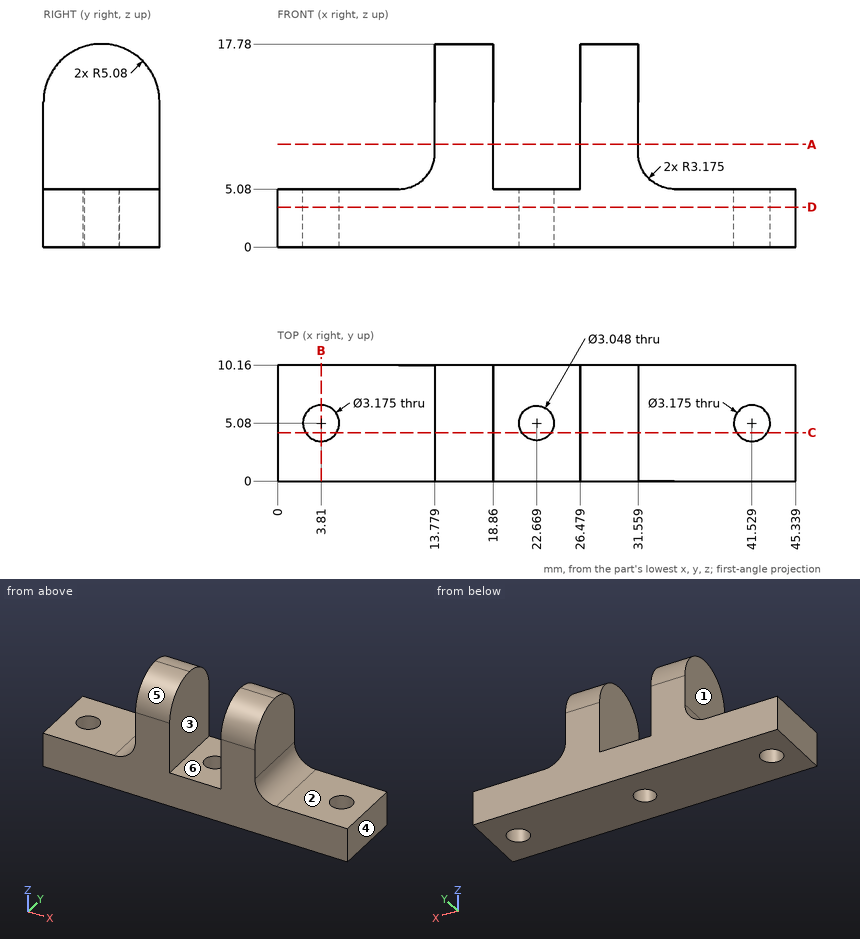
Here's the drawing with two shaded views (mm, measured from the low corner). I have some questions. A direction names the side the tool comes from. Give positions to 0.01 mm unless a question says otherwise; leave off trailing zeros. Loops run counter-clockwise (first coordinate to the right, second up) from the corner with the lowest first, then second, coordinate; pieces in that order, holes last. Notation, with made-up numbers: (2, -36.75) -> (48, -36.75) arc R11 cw to (48, -20.75) -> close; hole circle Ø1 at (-29, 67.25). An arc over 180 degrees is marked (long way). Answer as a JSON object with one key per item and string values. Group by question number.
Item 1: Imagine slicing it at C-C on y = 4.25. Give the number of separate pieces and of enclosed holes in the cut face.
Item 2: Thinking about a two-plate mould opening in X: for the marked faces 4, 5 and 6, which applies, pulls with the +X half, pulls with the -X half, needs draft (parallel to the pull), parting line crosses it, or undercut?
Item 3: I need wall thicknesses on L1, parallel to Y at x = 3.81, z = 3; L2, parallel to X at y = 6, z = 8; L3, parallel to X at y = 5.5, z = 3 (1 decimal). Which ranges of each line are inside material? Lowest first, please.
Item 4: Imagine slicing it at A-A on z = 9. Write out the boundary of the cut face in (x, y).
Item 5: Imagine slicing it at D-D on z = 3.5. Write out the boundary of the cut face in (x, y) (1 decimal).
Item 6: Will these pins go through, and if not, where does the flat tip stop? pin 1 (3.5 mm diameter, centred on x = 22.67, y = 5.08, fed in from +Z); pin 2 (5 mm diameter, centred on y = 6, z = 11.5, fed in from +X); pin 3 (6 mm diameter, centred on x = 26.5, y = 9, fed in from +Z).
Item 7: Imagine slicing it at B-B on x = 3.81. Write out the boundary of the cut face in (y, z).
Item 8: On a 3-axis mill with a long thin cutter (end or side, diameter ignored), from which of +Z, -Z, +X, -X, +Y, -Y can I reach the whole of each face in a straight line? I mean the marked faces 1, 2 and 3. Say none if no direction works.
Answer list:
{
 "1": {"separate pieces": "4", "enclosed holes": "0"},
 "2": {"face 4": "pulls with the +X half", "face 5": "needs draft", "face 6": "undercut"},
 "3": {"L1": "y = 0 to 3.49, 6.67 to 10.16", "L2": "x = 13.77 to 18.86, 26.48 to 31.57", "L3": "x = 0 to 2.3, 5.3 to 21.2, 24.1 to 40, 43.1 to 45.3"},
 "4": {"outline": "(13.78, 0) -> (18.86, 0) -> (18.86, 10.16) -> (13.78, 10.16) -> close; (26.48, 0) -> (31.56, 0) -> (31.56, 10.16) -> (26.48, 10.16) -> close"},
 "5": {"outline": "(0, 0) -> (45.3, 0) -> (45.3, 10.2) -> (0, 10.2) -> close; hole circle Ø3.2 at (3.8, 5.1); hole circle Ø3 at (22.7, 5.1); hole circle Ø3.2 at (41.5, 5.1)"},
 "6": {"pin 1": "stops at z = 5.08", "pin 2": "stops at x = 31.56", "pin 3": "stops at z = 17.7"},
 "7": {"outline": "(0, 0) -> (3.49, 0) -> (3.49, 5.08) -> (0, 5.08) -> close; (6.67, 0) -> (10.16, 0) -> (10.16, 5.08) -> (6.67, 5.08) -> close"},
 "8": {"face 1": "+Z, -X, +Y, -Y", "face 2": "+Z, +X, +Y, -Y", "face 3": "+Z, +Y, -Y"}
}
